from build123d import *

# Parameters (mm, degrees)
SKETCH3_R                  = 21
SKETCH3_R_2                = 11
BOSS_EXTRUDE1_DEPTH        = 14.3
SKETCH4_R                  = 21
SKETCH4_R_2                = 10
BOSS_EXTRUDE2_DEPTH        = 7
M4_TAPPED_HOLE1_AT_2_COUNT = 2
M4_TAPPED_HOLE1_AT_2_PITCH = 24.04163056
M4_TAPPED_HOLE1_AT_3_COUNT = 2
M4_TAPPED_HOLE1_AT_3_PITCH = 34
M4_TAPPED_HOLE1_AT_4_COUNT = 2
M4_TAPPED_HOLE1_AT_4_PITCH = 24.04163056
BOSS_EXTRUDE3_REACH        = 59.875
BOSS_EXTRUDE3_END_RADIUS   = 21
SKETCH7_W                  = 28.6
SKETCH7_H                  = 20
SKETCH11_W                 = 20
SKETCH11_H                 = 8
CUT_EXTRUDE2_DEPTH         = 10
SKETCH12_R                 = 2
CUT_EXTRUDE3_DEPTH         = 47.113880774
FILLET1_R                  = 15
FILLET5_R                  = 1
M8_TAPPED_HOLE1_D          = 6.8
M8_TAPPED_HOLE1_DEPTH      = 19.75
M8_TAPPED_HOLE1_TIP        = 2.042926105


with BuildPart() as part:
    # Sketch3 → Boss-Extrude1 (new body)
    with BuildSketch(Plane(origin=(0, 0, 0), x_dir=(0, 0, -1), z_dir=(1, 0, 0))):
        Circle(SKETCH3_R)
        Circle(SKETCH3_R_2, mode=Mode.SUBTRACT)
    boss_extrude1 = extrude(amount=BOSS_EXTRUDE1_DEPTH)

    # Sketch4 → Boss-Extrude2 (add)
    with BuildSketch(Plane(origin=(0, 0, 0), x_dir=(0, 0, -1), z_dir=(1, 0, 0))):
        Circle(SKETCH4_R)
        Circle(SKETCH4_R_2, mode=Mode.SUBTRACT)
    boss_extrude2 = extrude(amount=BOSS_EXTRUDE2_DEPTH)

    # Sketch15 → M4 Tapped Hole1 (revolve, cut)
    with BuildSketch(Plane(origin=(14.3, 17, 0), x_dir=(0, 0, -1), z_dir=(0, 1, 0))):
        Polygon((0, 0), (0, 8.991420021), (1.65, 8), (1.65, 0), align=None)
    m4_tapped_hole1 = revolve(axis=Axis((20.65, 17, 0), (-1, 0, 0)), mode=Mode.SUBTRACT)

    # M4 Tapped Hole1 at 2: M4 Tapped Hole1 ×2
    with Locations(*[Vector(0, -0.7071067811865479, -0.7071067811865472) * (i * M4_TAPPED_HOLE1_AT_2_PITCH) for i in range(1, M4_TAPPED_HOLE1_AT_2_COUNT)]):
        add(m4_tapped_hole1, mode=Mode.SUBTRACT)

    # M4 Tapped Hole1 at 3: M4 Tapped Hole1 ×2
    with Locations(*[(0, -i * M4_TAPPED_HOLE1_AT_3_PITCH, 0) for i in range(1, M4_TAPPED_HOLE1_AT_3_COUNT)]):
        add(m4_tapped_hole1, mode=Mode.SUBTRACT)

    # M4 Tapped Hole1 at 4: M4 Tapped Hole1 ×2
    with Locations(*[Vector(0, -0.7071067811865474, 0.7071067811865478) * (i * M4_TAPPED_HOLE1_AT_4_PITCH) for i in range(1, M4_TAPPED_HOLE1_AT_4_COUNT)]):
        add(m4_tapped_hole1, mode=Mode.SUBTRACT)

    # Mirror1: Boss-Extrude1, Boss-Extrude2, M4 Tapped Hole1 across plane
    add(boss_extrude1.mirror(Plane(origin=(0, 0, 0), x_dir=(0, 0, 1), z_dir=(1, 0, 0))))
    add(boss_extrude2.mirror(Plane(origin=(0, 0, 0), x_dir=(0, 0, 1), z_dir=(1, 0, 0))))
    add(m4_tapped_hole1.mirror(Plane(origin=(0, 0, 0), x_dir=(0, 0, 1), z_dir=(1, 0, 0))), mode=Mode.SUBTRACT)

    # Mirror1 copy 1 sketch → Mirror1 copy 1 (revolve, cut)
    with BuildSketch(Plane(origin=(-14.3, 0, -17), x_dir=(0, 0, -1), z_dir=(0, 1, 0))):
        Polygon((0, 0), (0, -8.991420021), (1.65, -8), (1.65, 0), align=None)
    revolve(axis=Axis((-20.65, 0, -17), (-1, 0, 0)), mode=Mode.SUBTRACT)

    # Mirror1 copy 2 sketch → Mirror1 copy 2 (revolve, cut)
    with BuildSketch(Plane(origin=(-14.3, -17, 0), x_dir=(0, 0, -1), z_dir=(0, 1, 0))):
        Polygon((0, 0), (0, -8.991420021), (1.65, -8), (1.65, 0), align=None)
    revolve(axis=Axis((-20.65, -17, 0), (-1, 0, 0)), mode=Mode.SUBTRACT)

    # Mirror1 copy 3 sketch → Mirror1 copy 3 (revolve, cut)
    with BuildSketch(Plane(origin=(-14.3, 0, 17), x_dir=(0, 0, -1), z_dir=(0, 1, 0))):
        Polygon((0, 0), (0, -8.991420021), (1.65, -8), (1.65, 0), align=None)
    revolve(axis=Axis((-20.65, 0, 17), (-1, 0, 0)), mode=Mode.SUBTRACT)

    # Boss-Extrude3: up to this cylinder (the profile starts outside it)
    boss_extrude3_end = Plane(origin=(0, 0, 0), z_dir=(-1, 0, 0)) * Cylinder(BOSS_EXTRUDE3_END_RADIUS, 162.75, mode=Mode.PRIVATE)
    # Sketch7 → Boss-Extrude3 (add, up to the surface)
    with BuildSketch(Plane.XY.offset(31), mode=Mode.PRIVATE) as boss_extrude3_sk1:
        Rectangle(SKETCH7_W, SKETCH7_H)
    boss_extrude3_tool1 = extrude(boss_extrude3_sk1.sketch, amount=-BOSS_EXTRUDE3_REACH, mode=Mode.PRIVATE) - boss_extrude3_end
    add(boss_extrude3_tool1.solids().sort_by_distance((0, 0, 31))[0])

    # Sketch11 → Cut-Extrude2 (cut)
    with BuildSketch(Plane.XY.offset(31)):
        Rectangle(SKETCH11_W, SKETCH11_H)
    extrude(amount=-CUT_EXTRUDE2_DEPTH, mode=Mode.SUBTRACT)

    # Sketch12 → Cut-Extrude3 (cut, through all)
    with BuildSketch(Plane(origin=(0, 10, 0), x_dir=(1, 0, 0), z_dir=(0, 1, 0))):
        with Locations(Location((0, -26, 0), (0, 0, 180))):
            Circle(SKETCH12_R)
    extrude(amount=-CUT_EXTRUDE3_DEPTH, mode=Mode.SUBTRACT)

    # Fillet1
    # the kernel refuses this fillet: 15 mm, written as the material it adds along each edge
    with BuildSketch(Plane(origin=(14.3, -10, 18.466185313), x_dir=(0, -0.8068579760983849, -0.5907454666829176), z_dir=(-1, 0, 0))) as fillet1_piece_1_section:
        with BuildLine():
            CenterArc((7.709210641, 14.862173982), FILLET1_R, 216.20992664, 46.01703687)
            Line((-4.393659, 6.000991981), (0, 0))
            ThreePointArc((0, 0), (2.840235499, 0.192956426), (5.680470999, 0))
        make_face()
    fillet1_piece_1 = extrude(amount=28.6, mode=Mode.PRIVATE)
    fillet1_piece_1 = fillet1_piece_1 - Plane(origin=(0, -10.967889591, 26), x_dir=(-1, 0, 0), z_dir=(0, 1, 0)) * Cylinder(2, 82, mode=Mode.PRIVATE)
    add(fillet1_piece_1)
    with BuildSketch(Plane(origin=(14.3, 10, 18.466185313), x_dir=(0, 0.8068579760983845, -0.5907454666829182), z_dir=(-1, 0, 0))) as fillet1_piece_2_section:
        with BuildLine():
            CenterArc((7.709210641, -14.862173982), FILLET1_R, 97.773036491, 46.01703687)
            Line((-4.393659, -6.000991981), (0, 0))
            ThreePointArc((0, 0), (2.840235499, -0.192956426), (5.680470999, 0))
        make_face()
    fillet1_piece_2 = extrude(amount=28.6, mode=Mode.PRIVATE)
    fillet1_piece_2 = fillet1_piece_2 - Plane(origin=(0, 10.967889591, 26), x_dir=(-1, 0, 0), z_dir=(0, 1, 0)) * Cylinder(2, 82, mode=Mode.PRIVATE)
    add(fillet1_piece_2)

    # Fillet5
    fillet5_edges = [part.edges().sort_by_distance(p)[0] for p in [
        (10, 0, 31),
        (0, 4, 31),
        (-10, 0, 31),
        (0, -4, 31),
    ]]
    fillet(fillet5_edges, radius=FILLET5_R)

    # M8 Tapped Hole1
    with Locations(Plane.XY.offset(21)):
        with Locations((0, 0)):
            Hole(M8_TAPPED_HOLE1_D / 2, depth=M8_TAPPED_HOLE1_DEPTH)
            with Locations((0, 0, -(M8_TAPPED_HOLE1_DEPTH + M8_TAPPED_HOLE1_TIP / 2))):  # 118° drill point
                Cone(0, M8_TAPPED_HOLE1_D / 2, M8_TAPPED_HOLE1_TIP, mode=Mode.SUBTRACT)


solid = part.part
Could you check a few things on this model? Use its own coordinates, in mm. A direction names the side the tool comes from. Round coordinates to 2 decimals unless told otherwise and drop trailing zeros. Order: outer loops, then holes, each group sorted by start corner. A loop starts at its lowest first (then second) coordinate and runs counter-clockwise, first axis right, second up.
Q1. Thinking about a two-plate mould opening in X: for faces 1 (the face through (-10, 0, 26)), 2 (the face through (10.356, -0.496, 15.426)), 3 (the face through (5.48, 16.72, 0.04)), which applies, released by +X, released by -X, zero draft, split by the parting line, or undercut?
Geometry says:
face 1: undercut
face 2: zero draft
face 3: released by +X
Q2. Which directions (+Z, -Z, +X, -X, +Y, -Y) give clear straight access to the entire face, cutting with the end or side of a thin tool? Please do faces 4 (the face through (-0.2, -10, 28.5)), 5 (the face through (-10.356, 15.364, 0.215)), 6 (the face through (-14.3, 0, 13)), 7 (the face through (10.356, -0.496, -18.574)), 8 (the face through (-0.1, -4, 23.6)).
Geometry says:
face 4: +Z, +X, -X, -Y
face 5: -X
face 6: +Z, -Z, -X, +Y, -Y
face 7: +X
face 8: +Z
Q3. Imagine slicing it at B-B, the plane y = 2.5. List the corners of the cut face in (x, z) for me, then the cut area to 3 significant figures.
Geometry says:
outline: (-14.3, -20.85) - (14.3, -20.85) - (14.3, -10.71) - (7, -10.71) - (7, -9.68) - (-7, -9.68) - (-7, -10.71) - (-14.3, -10.71) - close; (-14.3, 10.71) - (-7, 10.71) - (-7, 9.68) - (-2.3, 9.68) - (-2.3, 21) - (-10, 21) - (-10, 30) arc R1 ccw to (-11, 31) - (-14.3, 31) - close; (2.3, 9.68) - (7, 9.68) - (7, 10.71) - (14.3, 10.71) - (14.3, 31) - (11, 31) arc R1 ccw to (10, 30) - (10, 21) - (2.3, 21) - close
area: 646 mm2
Q4. Imagine slicing it at C-C, the plane y = 7. List the corners of the cut face in (x, z) for me, then the cut area to 3 significant figures.
Geometry says:
outline: (-14.3, -19.8) - (14.3, -19.8) - (14.3, -8.49) - (7, -8.49) - (7, -7.14) - (-7, -7.14) - (-7, -8.49) - (-14.3, -8.49) - close; (-14.3, 8.49) - (-7, 8.49) - (-7, 7.14) - (7, 7.14) - (7, 8.49) - (14.3, 8.49) - (14.3, 31) - (-14.3, 31) - close; hole circle Ø4 at (0, 26)
area: 993 mm2
Q5. Imagine slicing it at A-A, the plane y = -8. List the corners of the cut face in (x, z) for me, then the cut area to 3 significant figures.
Geometry says:
outline: (-14.3, -19.42) - (14.3, -19.42) - (14.3, -7.55) - (7, -7.55) - (7, -6) - (-7, -6) - (-7, -7.55) - (-14.3, -7.55) - close; (-14.3, 7.55) - (-7, 7.55) - (-7, 6) - (7, 6) - (7, 7.55) - (14.3, 7.55) - (14.3, 31) - (-14.3, 31) - close; hole circle Ø4 at (0, 26)
area: 1,040 mm2
Q6. Imagine slicing it at D-D, the plane z = -13. List the corners of the cut face in (x, y) for me, then the cut area to 3 significant figures.
Geometry says:
outline: (-14.3, -16.49) - (14.3, -16.49) - (14.3, 16.49) - (-14.3, 16.49) - close
area: 943 mm2
Q7. Please list where these lines run through material, in increasing order: probe 1 along Y at (x, z) = (11.25, 0); probe 2 along Y at (x, z) = (1.25, -0.5); probe 3 along X at (y, z) = (3, 23.5).
Geometry says:
probe 1: y = -21 to -18.65, -15.35 to -11, 11 to 15.35, 18.65 to 21
probe 2: y = -20.99 to -9.99, 9.99 to 20.99
probe 3: x = -14.3 to -10, 10 to 14.3
Q8. I'm going to push flat-ended pins straight in: P1, Ø2, axis at y = 17, z = 0, coming from the -X side; P2, Ø5.5, axis at x = 3.5, z = 28.5, coming from the -Y side; P3, Ø4, axis at x = -2.5, y = -0.5, coming from the +Z side. Where does each tip first touch, or does it pass through?
Geometry says:
P1: stops at x = -5.91
P2: stops at y = -10
P3: stops at z = 21
